The drawing under review shows one solid part. Ordinate dimensions are in mm from its lowest x, y, z. A direction names the side the tool comes from. Give positions to 0.01 mm unless a question says otherwise; leave off trailing zeros. Loops run counter-clockwise (first coordinate to the right, second up) from the corner with the lowest first, then second, coordinate; pieces in that order, holes last. Notation, with made-up numbers: (-15.5, 78) -> (-9.5, 78) arc R32 ccw to (-9.5, 114) -> close; hole circle Ø1 at (-25.5, 27.5). An arc over 180 degrees is marked (long way). Answer in a Markdown table with one row per item. Add a question column.
(1) For the marked faces 1 and 2, list the 3-axis set-ups (+Z, -Z, +X, -X, +Y, -Y) from which the entire face can be reached by the end or side of a thin tool; tool diameter is ignored.
(2) For pin 1 (2 mm diameter, centred on y = 3, z = 10, fed in from +X); pin 2 (6 mm diameter, centred on x = 23, z = 6.5, fed in from +Y), all flat-tipped, find the tip position at first contact; note any pin that passes through.
(3) Consider section D-D on z = 15. Write out the cut boundary in (x, y).
(4) For line 1 (Y direction, x = 8, z = 5.25); line 2 (X direction, y = 0.9, z = 10), list the stretches that pass through material, from the lowest coordinate up.
(5) Consider section C-C on y = 0.5. Write out the cut boundary in (x, z), then the cut area to 3 significant figures.
(6) Consider section A-A on x = 22.5. Write out the cut boundary in (y, z).
(7) Consider section B-B on z = 10. Write out the cut boundary in (x, y).
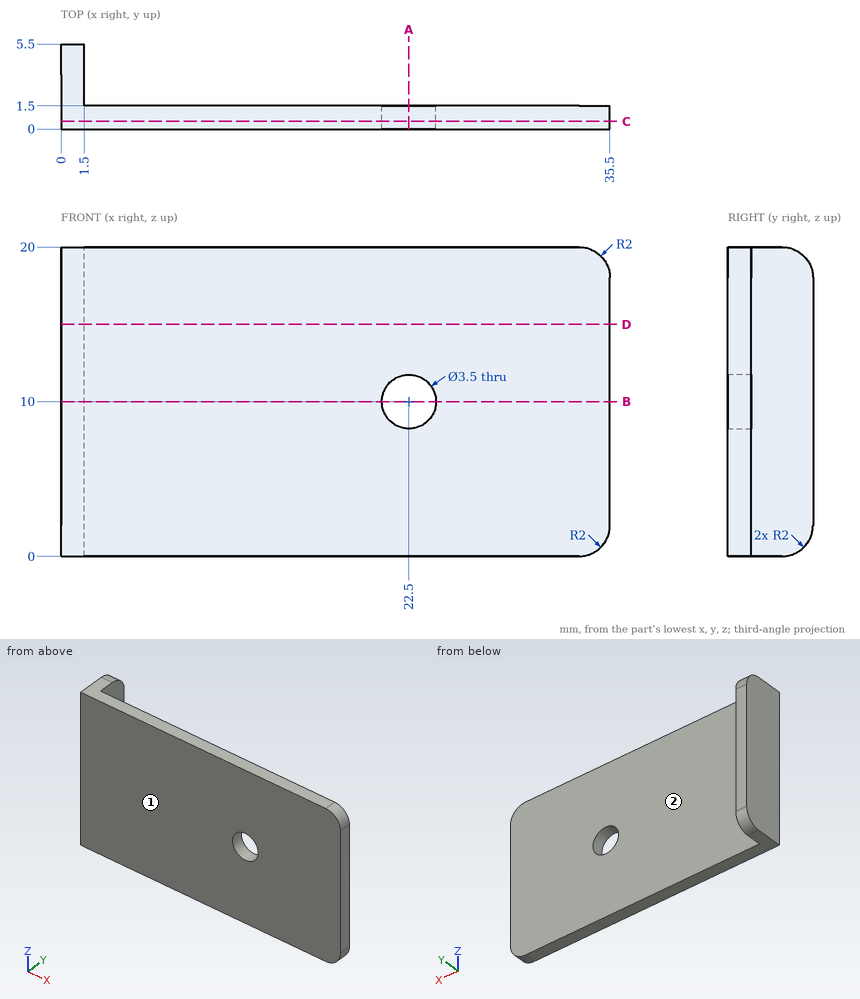
Values follow:
| question | item | result |
|---|---|---|
| 1 | face 1 | +Z, -Z, +X, -X, -Y |
| 1 | face 2 | +Z, -Z, +X, +Y |
| 2 | pin 1 | x = 1.5 |
| 2 | pin 2 | y = 1.5 |
| 3 | outline | (0, 0) -> (35.5, 0) -> (35.5, 1.5) -> (1.5, 1.5) -> (1.5, 5.5) -> (0, 5.5) -> close |
| 4 | line 1 | 0 to 1.5 |
| 4 | line 2 | 0 to 20.75, 24.25 to 35.5 |
| 5 | outline | (0, 0) -> (33.5, 0) arc R2 ccw to (35.5, 2) -> (35.5, 18) arc R2 ccw to (33.5, 20) -> (0, 20) -> close; hole circle Ø3.5 at (22.5, 10) |
| 5 | area | 699 mm2 |
| 6 | outline | (0, 0) -> (1.5, 0) -> (1.5, 8.25) -> (0, 8.25) -> close; (0, 11.75) -> (1.5, 11.75) -> (1.5, 20) -> (0, 20) -> close |
| 7 | outline | (0, 0) -> (20.75, 0) -> (20.75, 1.5) -> (1.5, 1.5) -> (1.5, 5.5) -> (0, 5.5) -> close; (24.25, 0) -> (35.5, 0) -> (35.5, 1.5) -> (24.25, 1.5) -> close |
